Input: part model. Units: mm. Frame: model coordinates. Coordinates: 2 decimals unless noted, no trailing zeros. Write each loop counter-clockwise with the first axis right and the second up, starting at its lowest first coordinate (ties: lowest second). Pieces come first, ordered by that corner, then holes. Notation, with made-up numbers: (75, 85.25) - (91, 85.25) arc R16 cw to (91, 113.25) - close; hole circle Ø1 at (-18.5, -15). An arc over 180 degrees is marked (long way). One line per question, with ' | ' between items. Start each with the question number.
1) Line query: line 1 (Z direction, x = 505, y = 0.3); line 2 (X direction, y = 0.8, z = -80); line 3 (X direction, y = 0.6, z = -112.5). Output: solid intervals per line, ascending.
2) Section query B-B on z = -122. Return loops of the section in (x, y).
3) Section query A-A on y = 0.75. Return loops of the section in (x, z).
4) First-contact query: P1, Ø0.8, axis at x = 534.5, y = 0.5, coming from the -Z side; P2, Ø4.5, axis at x = 505, z = -80, coming from the +Y side. Flat tips, straight axial feed; report the tip coordinate or a pass-through.
Autodesk Inventor part; units mm, degrees
ref_plane "YZ Plane" through (0, 0, 0) normal (1, 0, 0) x (0, 1, 0)
ref_plane "XZ Plane" through (0, 0, 0) normal (0, 1, 0) x (-1, 0, 0)
ref_plane "XY Plane" through (0, 0, 0) normal (0, 0, 1) x (1, 0, 0)
sketch "Sketch1" plane through (0, 0, 0) normal (0, 1, 0) x (-1, 0, 0)
  line L0 (0, 0) -> (-515, 0)
  line L1 (-515, 0) -> (-515, -150)
  line L2 (-515, -150) -> (0, -150)
  line L3 (0, -150) -> (0, 0)
  dimension "d0" = 515
  dimension "d1" = 150
extrude "Extrusion1" add sketch "Sketch1" along normal blind 1.6
sketch "Sketch2" plane through (0, 1.6, 0) normal (0, 1, 0) x (1, 0, 0)
  line L0 (515, 0) -> (495, 0)
  line L1 (495, 0) -> (495, 60)
  line L2 (495, 60) -> (515, 60)
  line L3 (515, 60) -> (515, 0)
  circle A0 centre (505, 80) radius 2.5
  circle A1 centre (505, 130) radius 2.5
  line L4 (515, 150) -> (0, 150)
  point P0 (0, 0)
  point P1 (505, 60)
  dimension "d6" = 20
  dimension "d7" = 60
  dimension "d10" = 5
  dimension "d11" = 5
  dimension "d12" = 50
  dimension "d13" = 20
extrude "Extrusion3" cut sketch "Sketch2" against normal blind 1.6
sketch "Sketch3" plane through (495, 1.6, 0) normal (1, 0, 0) x (0, 0, -1)
  line L0 (0, -1.6) -> (54, -1.6)
  line L1 (54, -1.6) -> (54, 0)
  line L2 (54, 0) -> (0, 0)
  line L3 (0, 0) -> (0, -1.6)
  dimension "d16" = 54
  dimension "d17" = 1.6
extrude "Extrusion4" add sketch "Sketch3" along normal blind 95
properties part number "X-Axis Panel Right" material "Steel"
Answer key:
1) line 1: -150 to -132.5, -127.5 to -82.5, -77.5 to -60, -54 to 0 | line 2: 0 to 502.5, 507.5 to 515 | line 3: 0 to 515
2) outline: (0, 0) - (515, 0) - (515, 1.6) - (0, 1.6) - close
3) outline: (0, -150) - (515, -150) - (515, -60) - (495, -60) - (495, -54) - (590, -54) - (590, 0) - (0, 0) - close; hole circle Ø5 at (505, -130); hole circle Ø5 at (505, -80)
4) P1: z = -54 | P2: through
